Can you work these out from the drawing? Everything is in mm from the part's minimum corner. Round coordinates to 2 decimals unless told otherwise and drop trailing zeros. Order: outer loops, then holes, each group sorted by start corner. A loop starts at its lowest first (then second) coordinate and runs counter-clockwise, first axis right, second up. Notation, with made-up numbers: M 2.25,49 L 45.25,49 A31 cw 45.25,81 Z; hole C -32,57 d1. An arc over 180 degrees is marked long. Write each question's results on one line, items separated by ' | '. Start each with the question number.
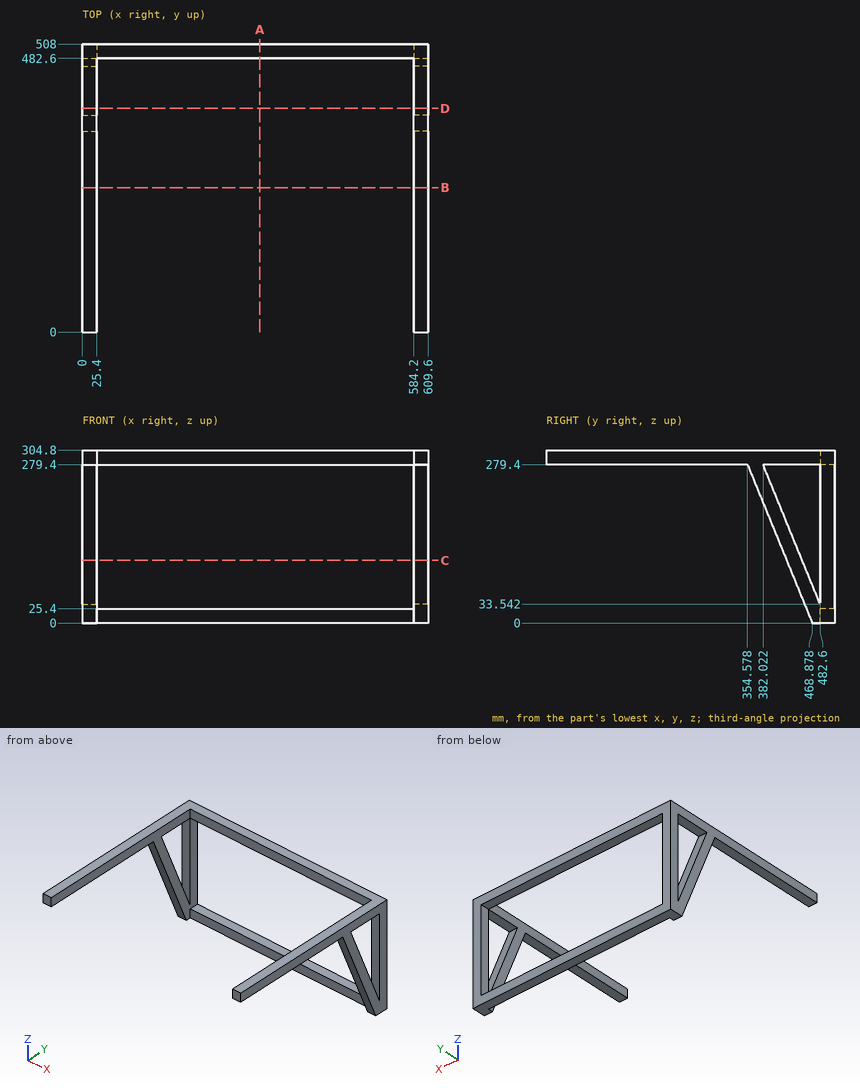
(1) I want a section at B-B on y = 255. Write out the boundary of the cut face in (x, z).
(2) I want a section at D-D on y = 394.5. Write out the boundary of the cut face in (x, z), and give its area (3 significant figures).
(3) I want a section at A-A on x = 312.5. Write out the boundary of the cut face in (y, z), and give its area (3 significant figures).
(4) Please list where these lines run through material, in increasing order: line 1 (X direction, y = 453, z = 75.5); line 2 (Y direction, x = 503, z = 282.5).
(5) I want a section at C-C on z = 110.5. Write out the boundary of the cut face in (x, y).
(6) I'm going to push flat-ended pins straight in: pin 1 Ø7.5 at (x, y) = (591, 231) entering from -Z; pin 2 Ø20.5 at (x, y) = (10, 446) entering from -Z; pin 3 Ø12.5 at (x, z) = (367.5, 290.5) entering from -Y. Where does each tip first touch, or does it pass through?
Solutions:
1) outline: M 0,279.4 L 25.4,279.4 L 25.4,304.8 L 0,304.8 Z; M 584.2,279.4 L 609.6,279.4 L 609.6,304.8 L 584.2,304.8 Z
2) outline: M 0,181.81 L 25.4,181.81 L 25.4,248.9 L 0,248.9 Z; M 0,279.4 L 25.4,279.4 L 25.4,304.8 L 0,304.8 Z; M 584.2,181.81 L 609.6,181.81 L 609.6,248.9 L 584.2,248.9 Z; M 584.2,279.4 L 609.6,279.4 L 609.6,304.8 L 584.2,304.8 Z | area: 4,700 mm^2
3) outline: M 482.6,0 L 508,0 L 508,25.4 L 482.6,25.4 Z; M 482.6,279.4 L 508,279.4 L 508,304.8 L 482.6,304.8 Z | area: 1,290 mm^2
4) line 1: 0 to 25.4, 584.2 to 609.6 | line 2: 482.6 to 508
5) outline: M 0,423.67 L 25.4,423.67 L 25.4,451.12 L 0,451.12 Z; M 0,482.6 L 25.4,482.6 L 25.4,508 L 0,508 Z; M 584.2,423.67 L 609.6,423.67 L 609.6,451.12 L 584.2,451.12 Z; M 584.2,482.6 L 609.6,482.6 L 609.6,508 L 584.2,508 Z
6) pin 1: z = 279.4 | pin 2: z = 30.87 | pin 3: y = 482.6
